Design review of the part built by this model. Coordinates are the model's own, in mm. A direction names the side the tool comes from. Coordinates: 2 decimals unless noted, no trailing zeros. Order: outer loops, then holes, each group sorted by start corner. A loop starts at its lowest first (then second) coordinate and runs counter-clockwise, first axis right, second up. Notation, with made-up numbers: (-28.5, 20.5) - (-9.5, 20.5) arc R22 ccw to (-9.5, 58.5) - close; hole circle Ø2 at (-7.75, 42.5). An arc over 180 degrees is marked (long way). Write each question's results on one line, items separated by ' | '. Start each with the question number.
```python
from build123d import *

# Parameters (mm, degrees)
SKETCH001_R             = 1.55
SKETCH001_R_2           = 0.6
PAD004_DEPTH            = 2.8
FILLET_R                = 0.4
FILLET001_R             = 5
SKETCH019_R             = 3.5
POCKET_DEPTH            = 2.801
BODY014_PLACEMENT_ANGLE = 180


with BuildPart() as part:
    # Sketch001 (on DatumPlane) → Pad004 (new body)
    with BuildSketch(Plane(origin=(-24.3, 0, 0), x_dir=(0, -1, 0), z_dir=(-1, 0, 0))):
        Polygon((-10, 84), (10, 84), (10, -53), (6, -53), (6, -50.2), (1.25, -50.2), (1.25, -47.2), (2.75, -47.2), (2.75, -44.7), (1.25, -44.7), (1.25, -37.7), (-1.25, -37.7), (-1.25, -44.7), (-2.75, -44.7), (-2.75, -47.2), (-1.25, -47.2), (-1.25, -50.2), (-6, -50.2), (-6, -53), (-10, -53), align=None)
        with Locations((0, -10)):
            Circle(SKETCH001_R, mode=Mode.SUBTRACT)
        with Locations((-7, 20)):
            Circle(SKETCH001_R_2, mode=Mode.SUBTRACT)
        with Locations((7, 20)):
            Circle(SKETCH001_R_2, mode=Mode.SUBTRACT)
        with BuildLine():
            ThreePointArc((3.1, 75), (0, 78.1), (-3.1, 75))
            Line((-3.1, 75), (-3.1, 50))
            ThreePointArc((-3.1, 50), (0, 46.9), (3.1, 50))
            Line((3.1, 50), (3.1, 75))
        make_face(mode=Mode.SUBTRACT)
    extrude(amount=PAD004_DEPTH)

    # Fillet
    fillet_edges = [part.edges().sort_by_distance(p)[0] for p in [
        (-25.7, 10, -53),
        (-25.7, 6, -53),
        (-25.7, -10, -53),
        (-25.7, -6, -53),
        (-25.7, 1.25, -50.2),
        (-25.7, -1.25, -50.2),
        (-25.7, 1.25, -37.7),
        (-25.7, -1.25, -37.7),
        (-25.7, 1.25, -47.2),
        (-25.7, -1.25, -47.2),
        (-25.7, 1.25, -44.7),
        (-25.7, -1.25, -44.7),
        (-25.7, -2.75, -47.2),
        (-25.7, 2.75, -47.2),
        (-25.7, 2.75, -44.7),
        (-25.7, -2.75, -44.7),
    ]]
    fillet(fillet_edges, radius=FILLET_R)

    # Fillet001
    fillet001_edges = [part.edges().sort_by_distance(p)[0] for p in [
        (-25.7, 10, 84),
        (-25.7, -10, 84),
    ]]
    fillet(fillet001_edges, radius=FILLET001_R)

    # Sketch019 (on Face47 of Fillet001) → Pocket (cut, through all)
    with BuildSketch(Plane(origin=(-27.1, 0, 0), x_dir=(0, -1, 0), z_dir=(-1, 0, 0))):
        Circle(SKETCH019_R)
    extrude(amount=-POCKET_DEPTH, mode=Mode.SUBTRACT)


with BuildPart() as part_1:
    # Body014 placement: moved
    add(part.part.moved(Location((0, 0, 20))).rotate(Axis((0, 0, 20), (0, 0, 1)), BODY014_PLACEMENT_ANGLE))


solid = part_1.part
```
(1) Take a section at A-A (z = 20). State the section outline as (x, y) points, plus the area to 3 significant figures.
(2) Tool access review of faces 1 (the face through (26, -6, -31)), 2 (the face through (25.7, -0.1, 66.9)), 3 (the face through (26, -10, 32)): name each direction out of +Z, -Z, +X, -X, +Y, -Y from which nothing blocks a thin tool from reaching the whole face with its end or side.
(3) Take a section at C-C (x = 25.45). State how many separate pieces and enclosed holes the cut face has, plus the area to 3 significant figures.
(4) To check wall thickness, follow line 1 along Y through (x, z) = (25.45, 40); line 2 along Z through (x, y) = (26.4, 0); line 3 along Y through (x, z) = (26.4, 80). State the ranges of each line that lie inside material, in increasing order. Write a range as [from, to].
(5) Take a section at B-B (z = 85.5). State the section outline as (x, y) points, plus the area to 3 significant figures.
(6) Clearance check with flat-ended pins moving along their axes: pin 1 (0.9 mm diameter, centred on x = 25.5, y = 0, fed in from -Z); pin 2 (0.6 mm diameter, centred on x = 25, y = 2, fed in from -Z); pin 3 (1.5 mm diameter, centred on x = 25, y = -7, fed in from +Z); pin 4 (1 mm diameter, centred on y = 7, z = 40, fed in from +X). State where each tip first meets the part, or that it passes through.
(7) Mouldability with a two-part tool opening along Y and no side actions: class faces 4 (the face through (26, -9, 102)), 5 (the face through (26, -4, -30.2)), 6 (the face through (26, 10, 34)), 7 (the face through (27.1, 0, 36)) as +Y half, -Y half, draft (parallel to the pull), parting line (faces both ways), or undercut.
Worked out:
1) outline: (24.3, -10) - (27.1, -10) - (27.1, -3.5) - (24.3, -3.5) - close; (24.3, 3.5) - (27.1, 3.5) - (27.1, 10) - (24.3, 10) - close | area: 36.4 mm^2
2) face 1: -Z, +X, -X | face 2: +X, -X | face 3: +Z, -Z, +X, -X, -Y
3) separate pieces: 1 | enclosed holes: 5 | area: 2,420 mm^2
4) line 1: [-10, -7.6], [-6.4, 6.4], [7.6, 10] | line 2: [-17.7, 8.45], [11.55, 16.5], [23.5, 66.9], [98.1, 104] | line 3: [-10, -3.1], [3.1, 10]
5) outline: (24.3, -10) - (27.1, -10) - (27.1, -3.1) - (24.3, -3.1) - close; (24.3, 3.1) - (27.1, 3.1) - (27.1, 10) - (24.3, 10) - close | area: 38.6 mm^2
6) pin 1: z = -17.7 | pin 2: z = -30.2 | pin 3: z = 103.84 | pin 4: through
7) face 4: -Y half | face 5: undercut | face 6: +Y half | face 7: draft
